```python
from build123d import *

# Parameters (mm, degrees)
SKETCH1_W           = 80
SKETCH1_H           = 100
BOSS_EXTRUDE1_DEPTH = 9
SKETCH2_W           = 68
SKETCH2_H           = 85.4
CUT_EXTRUDE1_DEPTH  = 7
SKETCH3_W           = 95
SKETCH3_H           = 115
SKETCH3_W_2         = 80
SKETCH3_H_2         = 100
BOSS_EXTRUDE2_DEPTH = 125
SKETCH6_W           = 95
SKETCH6_H           = 20
BOSS_EXTRUDE4_DEPTH = 3
SKETCH7_R           = 1.65
CUT_EXTRUDE2_DEPTH  = 10.5
SKETCH9_R           = 3
CUT_EXTRUDE3_DEPTH  = 3.2


with BuildPart() as part:
    # Sketch1 → Boss-Extrude1 (new body)
    with BuildSketch(Plane(origin=(0, 0, 0), x_dir=(1, 0, 0), z_dir=(0, 1, 0))):
        Rectangle(SKETCH1_W, SKETCH1_H)
    extrude(amount=BOSS_EXTRUDE1_DEPTH)

    # Sketch2 → Cut-Extrude1 (cut)
    with BuildSketch(Plane(origin=(0, 9, 0), x_dir=(1, 0, 0), z_dir=(0, 1, 0))):
        Rectangle(SKETCH2_W, SKETCH2_H)
    extrude(amount=-CUT_EXTRUDE1_DEPTH, mode=Mode.SUBTRACT)

    # Sketch3 → Boss-Extrude2 (add)
    with BuildSketch(Plane.XZ):
        Rectangle(SKETCH3_W, SKETCH3_H)
        Rectangle(SKETCH3_W_2, SKETCH3_H_2, mode=Mode.SUBTRACT)
    extrude(amount=-BOSS_EXTRUDE2_DEPTH)

    # Sketch6 → Boss-Extrude4 (add)
    with BuildSketch(Plane.XY.offset(57.5)):
        with Locations((0, 95)):
            Rectangle(SKETCH6_W, SKETCH6_H)
    extrude(amount=BOSS_EXTRUDE4_DEPTH)

    # Sketch7 → Cut-Extrude2 (cut)
    with BuildSketch(Plane.XY.offset(60.5)):
        with Locations((-11.5, 95)):
            Circle(SKETCH7_R)
        with Locations((11.5, 95)):
            Circle(SKETCH7_R)
    extrude(amount=-CUT_EXTRUDE2_DEPTH, mode=Mode.SUBTRACT)

    # Sketch9 → Cut-Extrude3 (cut)
    with BuildSketch(Plane(origin=(0, 0, 50), x_dir=(-1, 0, 0), z_dir=(0, 0, -1))):
        with Locations((-11.5, 95)):
            Circle(SKETCH9_R)
        with Locations((11.5, 95)):
            Circle(SKETCH9_R)
    extrude(amount=-CUT_EXTRUDE3_DEPTH, mode=Mode.SUBTRACT)


solid = part.part
```
For this review, take the finished solid that the model builds, in its own axes (mm). A direction names the side the tool comes from. Round coordinates to 2 decimals unless told otherwise and drop trailing zeros. Write each loop counter-clockwise with the first axis right and the second up, starting at its lowest first coordinate (ties: lowest second). Pieces come first, ordered by that corner, then holes. Notation, with made-up numbers: M 43.5,82 L 58.5,82 A16 cw 58.5,98 Z; hole C 37.5,1 d8. An arc over 180 degrees is marked long. One line per item, written item: value. Start each with the question number.
(1) Wall thickness on line 1 (X direction, y = 95, z = 58); line 2 (Y direction, x = 11.5, z = 57); line 3 (Y direction, x = -11.5, z = 52.4): over which ranges is each line inside the solid? List them lowest first.
(2) We need section A-A (y = 95). Give the boundary of the cut face in (x, z).
(3) Insertion check: pin 1 (6 mm diameter, centred on x = -3.5, y = 115, fed in from +Z); pin 2 (1 mm diameter, centred on x = -33, z = -25.5, fed in from +Y); pin 3 (1.5 mm diameter, centred on x = 4, z = 59, fed in from -Y); pin 4 (6 mm diameter, centred on x = 6.5, z = -43, fed in from -Y). Each pin has a flat end and moves straight along its axis. Give the tip position at first contact, or say it passes through.
(4) We need section C-C (x = 29). Give the boundary of the cut face in (y, z).
(5) The part is to be moulded in two halves that separate along Z. For faces 5 (the flat face through (-13, 94, 53.2)), 6 (the flat face through (-1, 95, 60.5)), 7 (the flat face through (-1, 105, 59)), say which applies: released by +Z, released by -Z, zero draft, split by the parting line, or undercut.
(6) We need section D-D (z = -47). Give the boundary of the cut face in (x, y), and give its area (4 significant figures).
(7) We need section B-B (x = 11.5). Give the boundary of the cut face in (y, z), and give its area (3 significant figures).
(8) Machinability: for faces 1 (the flat face through (-1, 42, 57.5)), 2 (the flat face through (-34, 6, 1)), 3 (the cylindrical face through (-10.85, 92.07, 51.58)), 4 (the cylindrical face through (11.1, 93.4, 56.9)), which of the approach directions +Z, -Z, +X, -X, +Y, -Y give a long, thin tool a straight path to every point of the face, cutting with its end or side? Answer none if there is none.
Result:
1. line 1: -47.5 to -13.15, -9.85 to 9.85, 13.15 to 47.5
1. line 2: 0 to 93.35, 96.65 to 125
1. line 3: 0 to 92, 98 to 125
2. outline: M -47.5,-57.5 L 47.5,-57.5 L 47.5,60.5 L 13.15,60.5 L 13.15,53.2 L 14.5,53.2 L 14.5,50 L 40,50 L 40,-50 L -40,-50 L -40,50 L -14.5,50 L -14.5,53.2 L -13.15,53.2 L -13.15,60.5 L -47.5,60.5 Z; M -9.85,53.2 L -8.5,53.2 L -8.5,50 L 8.5,50 L 8.5,53.2 L 9.85,53.2 L 9.85,60.5 L -9.85,60.5 Z
3. pin 1: z = 57.5
3. pin 2: y = 2
3. pin 3: y = 85
3. pin 4: y = 0
4. outline: M 0,-57.5 L 125,-57.5 L 125,-50 L 9,-50 L 9,-42.7 L 2,-42.7 L 2,42.7 L 9,42.7 L 9,50 L 125,50 L 125,57.5 L 105,57.5 L 105,60.5 L 85,60.5 L 85,57.5 L 0,57.5 Z
5. face 5: undercut
5. face 6: released by +Z
5. face 7: zero draft
6. outline: M -47.5,0 L 47.5,0 L 47.5,125 L 40,125 L 40,9 L -40,9 L -40,125 L -47.5,125 Z
6. area: 2,595 mm²
7. outline: M 0,-57.5 L 125,-57.5 L 125,-50 L 9,-50 L 9,-42.7 L 2,-42.7 L 2,42.7 L 9,42.7 L 9,50 L 92,50 L 92,53.2 L 93.35,53.2 L 93.35,60.5 L 85,60.5 L 85,57.5 L 0,57.5 Z; M 96.65,53.2 L 98,53.2 L 98,50 L 125,50 L 125,57.5 L 105,57.5 L 105,60.5 L 96.65,60.5 Z
7. area: 2,190 mm²
8. face 1: +Z, +X, -X, -Y
8. face 2: +Y
8. face 3: none
8. face 4: +Z
